Geometry: final body of the model. Coordinates: model frame, mm. Give positions to 0.01 mm unless a question says otherwise; leave off trailing zeros. Put each result on its own line as item: value. Start each with the question number.
1. First-contact query: P1, Ø4, axis at x = 0, z = 71.25, coming from the +Y side; P2, Ø1.8, axis at x = 47.38, z = -24.8, coming from the -Y side; P3, Ø0.8, axis at y = 1, z = 23, coming from the +X side; P4, Ø1, axis at x = 41, y = 1, coming from the +Z side. Flat tips, straight axial feed; report the tip coordinate or a pass-through.
2. Section A-A on y = 0.6. Count the separate pieces of the cut face and the enclosed holes in it, plus the area to 3 significant figures.
3. Ray query, line 1 along X through (y, z) = (1.5, -39.25); line 2 along X through (y, z) = (0.15, 20.5); line 3 along X through (y, z) = (1.1, 8). Return the intervals inside material, ascending. Write a range as from..to.
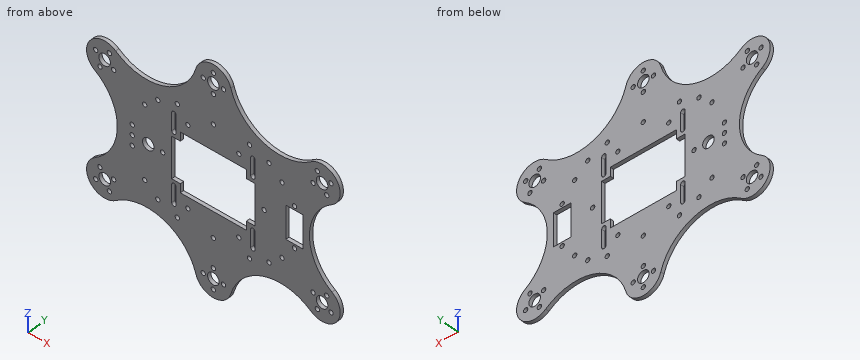
from build123d import *

# Parameters (mm, degrees)
SKETCH1_R           = 4
SKETCH1_R_2         = 1.5
SKETCH1_W           = 12
SKETCH1_H           = 22.5
BOSS_EXTRUDE1_DEPTH = 2.5


with BuildPart() as part:
    # Sketch1 → Boss-Extrude1 (new body)
    with BuildSketch(Plane(origin=(0, 0, 0), x_dir=(1, 0, 0), z_dir=(0, 1, 0))):
        with BuildLine():
            ThreePointArc((12.022120265, 67.673247628), (0, 76.75), (-12.022120265, 67.673247628))
            ThreePointArc((-12.022120265, 67.673247628), (-34.842613641, 43.81538777), (-67.414732932, 49.203285306))
            ThreePointArc((-67.414732932, 49.203285306), (-85.189938198, 46.45680917), (-81.819417269, 28.789306741))
            ThreePointArc((-81.819417269, 28.789306741), (-66.25, 0), (-81.819417269, -28.789306741))
            ThreePointArc((-81.819417269, -28.789306741), (-85.189938198, -46.45680917), (-67.414732932, -49.203285306))
            ThreePointArc((-67.414732932, -49.203285306), (-34.842613641, -43.81538777), (-12.022120265, -67.673247628))
            ThreePointArc((-12.022120265, -67.673247628), (0, -76.75), (12.022120265, -67.673247628))
            ThreePointArc((12.022120265, -67.673247628), (34.842613641, -43.81538777), (67.414732932, -49.203285306))
            ThreePointArc((67.414732932, -49.203285306), (85.189938198, -46.45680917), (81.819417269, -28.789306741))
            ThreePointArc((81.819417269, -28.789306741), (66.25, 0), (81.819417269, 28.789306741))
            ThreePointArc((81.819417269, 28.789306741), (85.189938198, 46.45680917), (67.414732932, 49.203285306))
            ThreePointArc((67.414732932, 49.203285306), (34.842613641, 43.81538777), (12.022120265, 67.673247628))
        make_face()
        with Locations(Location((0, 64.25, 0), (0, 0, 270))):
            Circle(SKETCH1_R, mode=Mode.SUBTRACT)
        with Locations(Location((-7, 64.25, 0), (0, 0, 270))):
            Circle(SKETCH1_R_2, mode=Mode.SUBTRACT)
        with Locations(Location((0, 57.25, 0), (0, 0, 270))):
            Circle(SKETCH1_R_2, mode=Mode.SUBTRACT)
        with Locations(Location((7, 64.25, 0), (0, 0, 270))):
            Circle(SKETCH1_R_2, mode=Mode.SUBTRACT)
        with Locations(Location((0, 71.25, 0), (0, 0, 270))):
            Circle(SKETCH1_R_2, mode=Mode.SUBTRACT)
        with Locations(Location((0, 37.375, 0), (0, 0, 270))):
            Circle(SKETCH1_R_2, mode=Mode.SUBTRACT)
        with Locations(Location((17.575, 27.5, 0), (0, 0, 270))):
            Circle(SKETCH1_R_2, mode=Mode.SUBTRACT)
        with Locations(Location((24.9, 37.375, 0), (0, 0, 270))):
            Circle(SKETCH1_R_2, mode=Mode.SUBTRACT)
        with Locations(Location((38.375, 32.75, 0), (0, 0, 270))):
            Circle(SKETCH1_R_2, mode=Mode.SUBTRACT)
        with Locations(Location((47.375, 24.800648389, 0), (0, 0, 270))):
            Circle(SKETCH1_R_2, mode=Mode.SUBTRACT)
        with Locations(Location((74.976618386, 39.25, 0), (0, 0, 270))):
            Circle(SKETCH1_R, mode=Mode.SUBTRACT)
        with Locations(Location((68.775, 36.003474258, 0), (0, 0, 270))):
            Circle(SKETCH1_R_2, mode=Mode.SUBTRACT)
        with Locations(Location((71.730092644, 45.451618386, 0), (0, 0, 270))):
            Circle(SKETCH1_R_2, mode=Mode.SUBTRACT)
        with Locations(Location((81.178236772, 42.496525742, 0), (0, 0, 270))):
            Circle(SKETCH1_R_2, mode=Mode.SUBTRACT)
        with Locations(Location((78.223144128, 33.048381614, 0), (0, 0, 270))):
            Circle(SKETCH1_R_2, mode=Mode.SUBTRACT)
        with Locations(Location((35, 0, 0), (0, 0, 270))):
            Circle(SKETCH1_R_2, mode=Mode.SUBTRACT)
        with Locations(Location((-35, 0, 0), (0, 0, 270))):
            Circle(SKETCH1_R_2, mode=Mode.SUBTRACT)
        with Locations(Location((-47.375, 24.800648389, 0), (0, 0, 270))):
            Circle(SKETCH1_R_2, mode=Mode.SUBTRACT)
        with Locations(Location((-38.375, 32.75, 0), (0, 0, 270))):
            Circle(SKETCH1_R_2, mode=Mode.SUBTRACT)
        with Locations(Location((-17.575, 27.5, 0), (0, 0, 270))):
            Circle(SKETCH1_R_2, mode=Mode.SUBTRACT)
        with Locations(Location((-24.9, 37.375, 0), (0, 0, 270))):
            Circle(SKETCH1_R_2, mode=Mode.SUBTRACT)
        with Locations(Location((-78.223144128, 33.048381614, 0), (0, 0, 270))):
            Circle(SKETCH1_R_2, mode=Mode.SUBTRACT)
        with Locations(Location((-81.178236772, 42.496525742, 0), (0, 0, 270))):
            Circle(SKETCH1_R_2, mode=Mode.SUBTRACT)
        with Locations(Location((-71.730092644, 45.451618386, 0), (0, 0, 270))):
            Circle(SKETCH1_R_2, mode=Mode.SUBTRACT)
        with Locations(Location((-68.775, 36.003474258, 0), (0, 0, 270))):
            Circle(SKETCH1_R_2, mode=Mode.SUBTRACT)
        with Locations(Location((-74.976618386, 39.25, 0), (0, 0, 270))):
            Circle(SKETCH1_R, mode=Mode.SUBTRACT)
        with Locations(Location((-24.9, -37.375, 0), (0, 0, 270))):
            Circle(SKETCH1_R_2, mode=Mode.SUBTRACT)
        with Locations(Location((-17.575, -27.5, 0), (0, 0, 270))):
            Circle(SKETCH1_R_2, mode=Mode.SUBTRACT)
        with Locations(Location((-38.375, -32.75, 0), (0, 0, 270))):
            Circle(SKETCH1_R_2, mode=Mode.SUBTRACT)
        with Locations(Location((-47.375, -24.800648389, 0), (0, 0, 270))):
            Circle(SKETCH1_R_2, mode=Mode.SUBTRACT)
        with Locations(Location((47.375, -24.800648389, 0), (0, 0, 270))):
            Circle(SKETCH1_R_2, mode=Mode.SUBTRACT)
        with Locations(Location((38.375, -32.75, 0), (0, 0, 270))):
            Circle(SKETCH1_R_2, mode=Mode.SUBTRACT)
        with Locations(Location((24.9, -37.375, 0), (0, 0, 270))):
            Circle(SKETCH1_R_2, mode=Mode.SUBTRACT)
        with Locations(Location((17.575, -27.5, 0), (0, 0, 270))):
            Circle(SKETCH1_R_2, mode=Mode.SUBTRACT)
        with Locations(Location((0, -37.375, 0), (0, 0, 270))):
            Circle(SKETCH1_R_2, mode=Mode.SUBTRACT)
        with Locations(Location((0, -71.25, 0), (0, 0, 270))):
            Circle(SKETCH1_R_2, mode=Mode.SUBTRACT)
        with Locations(Location((7, -64.25, 0), (0, 0, 270))):
            Circle(SKETCH1_R_2, mode=Mode.SUBTRACT)
        with Locations(Location((0, -57.25, 0), (0, 0, 270))):
            Circle(SKETCH1_R_2, mode=Mode.SUBTRACT)
        with Locations(Location((-7, -64.25, 0), (0, 0, 270))):
            Circle(SKETCH1_R_2, mode=Mode.SUBTRACT)
        with Locations(Location((0, -64.25, 0), (0, 0, 270))):
            Circle(SKETCH1_R, mode=Mode.SUBTRACT)
        with Locations(Location((78.223144128, -33.048381614, 0), (0, 0, 270))):
            Circle(SKETCH1_R_2, mode=Mode.SUBTRACT)
        with Locations(Location((81.178236772, -42.496525742, 0), (0, 0, 270))):
            Circle(SKETCH1_R_2, mode=Mode.SUBTRACT)
        with Locations(Location((71.730092644, -45.451618386, 0), (0, 0, 270))):
            Circle(SKETCH1_R_2, mode=Mode.SUBTRACT)
        with Locations(Location((68.775, -36.003474258, 0), (0, 0, 270))):
            Circle(SKETCH1_R_2, mode=Mode.SUBTRACT)
        with Locations(Location((74.976618386, -39.25, 0), (0, 0, 270))):
            Circle(SKETCH1_R, mode=Mode.SUBTRACT)
        with Locations(Location((-74.976618386, -39.25, 0), (0, 0, 270))):
            Circle(SKETCH1_R, mode=Mode.SUBTRACT)
        with Locations(Location((-68.775, -36.003474258, 0), (0, 0, 270))):
            Circle(SKETCH1_R_2, mode=Mode.SUBTRACT)
        with Locations(Location((-71.730092644, -45.451618386, 0), (0, 0, 270))):
            Circle(SKETCH1_R_2, mode=Mode.SUBTRACT)
        with Locations(Location((-81.178236772, -42.496525742, 0), (0, 0, 270))):
            Circle(SKETCH1_R_2, mode=Mode.SUBTRACT)
        with Locations(Location((-78.223144128, -33.048381614, 0), (0, 0, 270))):
            Circle(SKETCH1_R_2, mode=Mode.SUBTRACT)
        with Locations(Location((56, 13.875, 0), (0, 0, 270))):
            Circle(SKETCH1_R_2, mode=Mode.SUBTRACT)
        with Locations(Location((56, -13.875, 0), (0, 0, 270))):
            Circle(SKETCH1_R_2, mode=Mode.SUBTRACT)
        with Locations(Location((-44.9, 0, 0), (0, 0, 270))):
            Circle(SKETCH1_R, mode=Mode.SUBTRACT)
        with Locations(Location((-55.95, 0, 0), (0, 0, 270))):
            Circle(SKETCH1_R_2, mode=Mode.SUBTRACT)
        with Locations(Location((-55.95, 6.875, 0), (0, 0, 270))):
            Circle(SKETCH1_R_2, mode=Mode.SUBTRACT)
        with Locations(Location((-55.95, -6.875, 0), (0, 0, 270))):
            Circle(SKETCH1_R_2, mode=Mode.SUBTRACT)
        with BuildLine():
            Line((25.75, 17.65), (25.75, 29.65))
            ThreePointArc((25.75, 29.65), (27.25, 31.15), (28.75, 29.65))
            Line((28.75, 29.65), (28.75, 17.65))
            ThreePointArc((28.75, 17.65), (27.25, 16.15), (25.75, 17.65))
        make_face(mode=Mode.SUBTRACT)
        Polygon((-22.75, 20), (-22.75, 14), (-28.75, 14), (-28.75, -14), (-22.75, -14), (-22.75, -20), (22.75, -20), (22.75, -14), (28.75, -14), (28.75, 14), (22.75, 14), (22.75, 20), align=None, mode=Mode.SUBTRACT)
        with BuildLine():
            Line((-25.75, 17.65), (-25.75, 29.65))
            ThreePointArc((-25.75, 29.65), (-27.25, 31.15), (-28.75, 29.65))
            Line((-28.75, 29.65), (-28.75, 17.65))
            ThreePointArc((-28.75, 17.65), (-27.25, 16.15), (-25.75, 17.65))
        make_face(mode=Mode.SUBTRACT)
        with BuildLine():
            Line((-25.75, -17.65), (-25.75, -29.65))
            ThreePointArc((-25.75, -29.65), (-27.25, -31.15), (-28.75, -29.65))
            Line((-28.75, -29.65), (-28.75, -17.65))
            ThreePointArc((-28.75, -17.65), (-27.25, -16.15), (-25.75, -17.65))
        make_face(mode=Mode.SUBTRACT)
        with BuildLine():
            Line((25.75, -17.65), (25.75, -29.65))
            ThreePointArc((25.75, -29.65), (27.25, -31.15), (28.75, -29.65))
            Line((28.75, -29.65), (28.75, -17.65))
            ThreePointArc((28.75, -17.65), (27.25, -16.15), (25.75, -17.65))
        make_face(mode=Mode.SUBTRACT)
        with Locations((56, 0)):
            Rectangle(SKETCH1_W, SKETCH1_H, mode=Mode.SUBTRACT)
    extrude(amount=BOSS_EXTRUDE1_DEPTH)


solid = part.part
Resolved:
1. P1: y = 2.5
1. P2: through
1. P3: x = 75.43
1. P4: z = 42.43
2. separate pieces: 1
2. enclosed holes: 62
2. area: 12,700 mm^2
3. line 1: -87.48..-78.98, -70.98..70.98, 78.98..87.48
3. line 2: -73.03..-28.75, -25.75..25.75, 28.75..73.03
3. line 3: -67.19..-56.94, -54.96..-28.75, 28.75..50, 62..67.19
